```python
from build123d import *

# Parameters (mm, degrees)
SCHIZZO1_R                   = 20
ESTRUSIONE_ESTRUSIONE1_DEPTH = 10
SCHIZZO2_R                   = 10
TAGLIO_ESTRUSIONE1_DEPTH     = 10
RIPETIZIONECIRCOLARE1_DEPTH  = 10
TAGLIO_ESTRUSIONE2_DEPTH     = 6


# Read off the part's stored shape, not the designer's step: RipetizioneCircolare1
with BuildPart() as part:
    # Schizzo1 → Estrusione-Estrusione1 (new body)
    with BuildSketch(Plane(origin=(0, 0, 0), x_dir=(1, 0, 0), z_dir=(0, 1, 0))):
        with Locations(Location((0, 0, 0), (0, 0, 270))):
            Circle(SCHIZZO1_R)
    extrude(amount=ESTRUSIONE_ESTRUSIONE1_DEPTH)

    # Schizzo2 → Taglio-Estrusione1 (cut)
    with BuildSketch(Plane(origin=(0, 10, 0), x_dir=(1, 0, 0), z_dir=(0, 1, 0))):
        with Locations((0, 27)):
            Circle(SCHIZZO2_R)
    extrude(amount=-TAGLIO_ESTRUSIONE1_DEPTH, mode=Mode.SUBTRACT)

    # RipetizioneCircolare1 outline → RipetizioneCircolare1 (cut)
    with BuildSketch(Plane(origin=(0, 0, 0), x_dir=(1, 0, 0), z_dir=(0, 1, 0))):
        with BuildLine():
            ThreePointArc((-13.465911046, 14.787469009), (-17.320508076, 10), (-19.539279343, 4.268086546))
            ThreePointArc((-19.539279343, 4.268086546), (-14.722431864, 8.5), (-13.465911046, 14.787469009))
        make_face()
        with BuildLine():
            ThreePointArc((13.465911046, 14.787469009), (14.722431864, 8.5), (19.539279343, 4.268086546))
            ThreePointArc((19.539279343, 4.268086546), (17.320508076, 10), (13.465911046, 14.787469009))
        make_face()
        with BuildLine():
            ThreePointArc((19.539279343, -4.268086546), (14.722431864, -8.5), (13.465911046, -14.787469009))
            ThreePointArc((13.465911046, -14.787469009), (17.320508076, -10), (19.539279343, -4.268086546))
        make_face()
        with BuildLine():
            ThreePointArc((6.073368297, -19.055555556), (0, -17), (-6.073368297, -19.055555556))
            ThreePointArc((-6.073368297, -19.055555556), (0, -20), (6.073368297, -19.055555556))
        make_face()
        with BuildLine():
            ThreePointArc((-13.465911046, -14.787469009), (-14.722431864, -8.5), (-19.539279343, -4.268086546))
            ThreePointArc((-19.539279343, -4.268086546), (-17.320508076, -10), (-13.465911046, -14.787469009))
        make_face()
    extrude(amount=RIPETIZIONECIRCOLARE1_DEPTH, mode=Mode.SUBTRACT)

    # Schizzo3 → Taglio-Estrusione2 (cut)
    with BuildSketch(Plane.XZ):
        Polygon((0, 2), (-1.732050808, 1), (-1.732050808, -1), (0, -2), (1.732050808, -1), (1.732050808, 1), align=None)
    extrude(amount=-TAGLIO_ESTRUSIONE2_DEPTH, mode=Mode.SUBTRACT)


solid = part.part
```
CAD build for the part. Positions are in the model's coordinates, mm. A direction names the side the tool comes from. Coordinates: 2 decimals unless noted, no trailing zeros. Order: outer loops, then holes, each group sorted by start corner. A loop starts at its lowest first (then second) coordinate and runs counter-clockwise, first axis right, second up. Notation, with made-up numbers: (18.25, -28) - (27.25, -28) arc R19 cw to (27.25, -18) - close; hole circle Ø7 at (69.25, -31.5). An arc over 180 degrees is marked (long way). Use a Markdown table: item, result. Add a question column.
(1) Drill centre lines: line 1 along Z through (x, y) = (-5, 4.5); line 2 along Z through (x, y) = (-10, 9); line 3 along X through (y, z) = (8.5, -10.5). Where is each one in solid material? Low to high. Write a range as [from, to].
(2) Pull direction X, two halves, no side cores. Call faces 1 (the face through (20, 5, 0)), 2 (the face through (-0.85, 2.96, 1.51)), 3 (the face through (-14.677, 4.93, 8.579)): +X half, -X half, draft (parallel to the pull), parting line (faces both ways), or undercut.
(3) Which spindle directions (+Z, -Z, +X, -X, +Y, -Y) get a long thin tool onto all of the face, cutting with end or side? Do faces 4 (the face through (-9.95, 4.93, -17.35)), 5 (the face through (14.77, 4.93, 8.42)), 6 (the face through (-0.88, 2.96, -1.49)). Say none if no direction does.
(4) Saw through at D-D (x = 11). Give the cut face in (y, z).
(5) Saw through at B-B (y = 6.5). Give the cut face in (x, z), then the cut area to 3 significant figures.
(6) Flat gauge pins, fed straight in: pin 1 (1.5 mm diameter, centred on x = 0.5, y = 6.5, fed in from +Z); pin 2 (2 mm diameter, centred on x = -12.5, y = 7, fed in from +Z); pin 3 (1.5 mm diameter, centred on x = -4, y = 4, fed in from -Z). Where does each tip first touch, or does it go through?
(7) Saw through at A-A (y = 4.5). Give the cut face in (x, z), then the cut area to 3 significant figures.
(8) Saw through at C-C (z = 16). Give the cut face in (x, y), then the cut area to 3 significant figures.
Solved:
| question | item | result |
|---|---|---|
| 1 | line 1 | z = [-18.34, 18.34] |
| 1 | line 2 | z = [-17.32, 17.32] |
| 1 | line 3 | x = [-13.84, 13.84] |
| 2 | face 1 | +X half |
| 2 | face 2 | undercut |
| 2 | face 3 | -X half |
| 3 | face 4 | -Z, -X, +Y, -Y |
| 3 | face 5 | +X, +Y, -Y |
| 3 | face 6 | -Y |
| 4 | outline | (0, -16.7) - (10, -16.7) - (10, 16.7) - (0, 16.7) - close |
| 5 | outline | (-19.54, -4.27) arc R10 cw to (-13.47, -14.79) arc R20 ccw to (-6.07, -19.06) arc R10 cw to (6.07, -19.06) arc R20 ccw to (13.47, -14.79) arc R10 cw to (19.54, -4.27) arc R20 ccw to (19.54, 4.27) arc R10 cw to (13.47, 14.79) arc R20 ccw to (6.07, 19.06) arc R10 cw to (-6.07, 19.06) arc R20 ccw to (-13.47, 14.79) arc R10 cw to (-19.54, 4.27) arc R20 ccw to start |
| 5 | area | 1,110 mm² |
| 6 | pin 1 | stops at z = 17.08 |
| 6 | pin 2 | stops at z = 16.36 |
| 6 | pin 3 | stops at z = -18.2 |
| 7 | outline | (-19.54, -4.27) arc R10 cw to (-13.47, -14.79) arc R20 ccw to (-6.07, -19.06) arc R10 cw to (6.07, -19.06) arc R20 ccw to (13.47, -14.79) arc R10 cw to (19.54, -4.27) arc R20 ccw to (19.54, 4.27) arc R10 cw to (13.47, 14.79) arc R20 ccw to (6.07, 19.06) arc R10 cw to (-6.07, 19.06) arc R20 ccw to (-13.47, 14.79) arc R10 cw to (-19.54, 4.27) arc R20 ccw to start; hole (-1.73, -1) - (0, -2) - (1.73, -1) - (1.73, 1) - (0, 2) - (-1.73, 1) - close |
| 7 | area | 1,100 mm² |
| 8 | outline | (-12, 0) - (12, 0) - (12, 10) - (-12, 10) - close |
| 8 | area | 240 mm² |
